For this review, take the finished solid that the model builds, in its own axes (mm). Face numbers are marked on the shaded views. Coordinates: 2 decimals unless noted, no trailing zeros. Write each loop counter-clockwise with the first axis right and the second up, starting at its lowest first coordinate (ties: lowest second). Pieces come first, ordered by that corner, then holes.
1) To check wall thickness, follow line 1 along Z through (x, y) = (-60.9, 18); line 2 along X through (y, z) = (23, -2.5); line 3 along X through (y, z) = (-1, -20). State the ranges of each line that lie inside material, in increasing order.
2) We need section D-D on y = 45.5. Write out the cut boundary in (x, z), then the cut area to 3 significant figures.
3) We need section B-B on z = 20. Write out the cut boundary in (x, y).
4) We need section C-C on y = 6.5. Write out the cut boundary in (x, z), then the cut area to 3 significant figures.
5) We need section A-A on x = 45. Write out the cut boundary in (y, z), then the cut area to 4 significant figures.
6) Mouldability with a two-part tool opening along X and no side actions: class the marked faces 1, 2, 3 and 4 as pulls with the +X half, pulls with the -X half, needs draft (parallel to the pull), parting line crosses it, or undercut.
7) Insertion check: P1, Ø3, axis at x = -32.5, z = -2.5, coming from the +Y side; P2, Ø4, axis at y = 18, z = 20, coming from the -X side; P3, Ø2.5, axis at x = -61, z = 10, coming from the +Y side. Each pin has a flat end and moves straight along its axis. Give the tip position at first contact, or say it passes through.
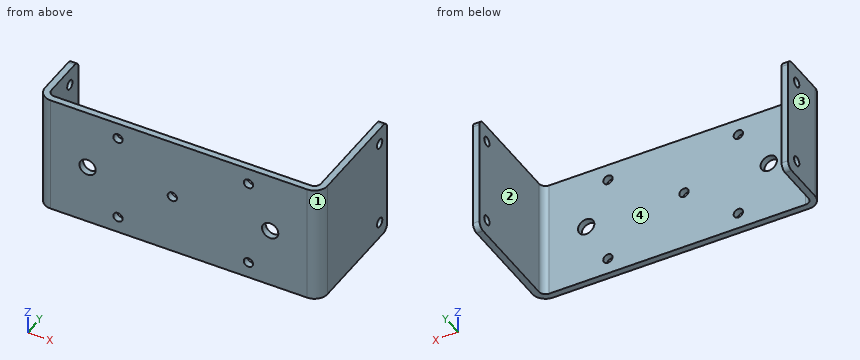
from build123d import *

# Parameters (mm, degrees)
SKETCH1_W                    = 124
SKETCH1_H                    = 55
SKETCH1_R                    = 1
SKETCH1_R_2                  = 3.75
BASE_FLANGE1_DEPTH           = 3
EDGE_FLANGE1_STRIP_W         = 18
EDGE_FLANGE1_STRIP_H         = 3
EDGE_FLANGE1_STRIP_CUT_DEPTH = 55
EDGE_FLANGE1_DEPTH           = 55
EDGE_FLANGE1_START           = 3
EDGE_FLANGE1_PROFILE_W       = 55
EDGE_FLANGE1_PROFILE_H       = 22
EDGE_FLANGE1_PROFILE_R       = 1
EDGE_FLANGE1_FLAT_DEPTH      = 3
EDGE_FLANGE2_STRIP_W         = 18
EDGE_FLANGE2_STRIP_H         = 3
EDGE_FLANGE2_STRIP_CUT_DEPTH = 55
EDGE_FLANGE2_DEPTH           = 55
EDGE_FLANGE2_START           = 3
EDGE_FLANGE2_PROFILE_W       = 55
EDGE_FLANGE2_PROFILE_H       = 48.5
EDGE_FLANGE2_PROFILE_R       = 1
EDGE_FLANGE2_FLAT_DEPTH      = 3
M4_CLEARANCE_HOLE1_D         = 4.3
M4_CLEARANCE_HOLE1_DEPTH     = 130
M4_CLEARANCE_HOLE2_D         = 4.3
M4_CLEARANCE_HOLE2_DEPTH     = 3
M4_CLEARANCE_HOLE2_TIP       = 1.291850331
M4_CLEARANCE_HOLE3_D         = 4.3
M4_CLEARANCE_HOLE3_DEPTH     = 3
M4_CLEARANCE_HOLE3_TIP       = 1.291850331
FILLET1_R                    = 3


# Sheet-metal steps are written as plain solids
with BuildPart() as part:
    # Sketch1 → Base-Flange1 (new body)
    with BuildSketch(Plane(origin=(0, 0, 0), x_dir=(1, 0, 0), z_dir=(0, 1, 0))):
        with Locations((3, 0)):
            Rectangle(SKETCH1_W, SKETCH1_H)
        with Locations(Location((-25, 20, 0), (0, 0, 270))):
            Circle(SKETCH1_R, mode=Mode.SUBTRACT)
        with Locations(Location((35, 20, 0), (0, 0, 270))):
            Circle(SKETCH1_R, mode=Mode.SUBTRACT)
        with Locations(Location((-25, -20, 0), (0, 0, 270))):
            Circle(SKETCH1_R, mode=Mode.SUBTRACT)
        with Locations(Location((35, -20, 0), (0, 0, 270))):
            Circle(SKETCH1_R, mode=Mode.SUBTRACT)
        with Locations(Location((45, 0, 0), (0, 0, 270))):
            Circle(SKETCH1_R_2, mode=Mode.SUBTRACT)
        with Locations(Location((-39, 0, 0), (0, 0, 270))):
            Circle(SKETCH1_R_2, mode=Mode.SUBTRACT)
        with Locations(Location((0, 0, 0), (0, 0, 270))):
            Circle(SKETCH1_R, mode=Mode.SUBTRACT)
    extrude(amount=-BASE_FLANGE1_DEPTH)

    # Edge-Flange1 strip (across the edge) → Edge-Flange1 strip cut (cut)
    with BuildSketch(Plane(origin=(-59, 0, -27.5), x_dir=(1, 0, 0), z_dir=(0, 0, 1))):
        with Locations((-6, -1.5)):
            Rectangle(EDGE_FLANGE1_STRIP_W, EDGE_FLANGE1_STRIP_H)
    extrude(amount=EDGE_FLANGE1_STRIP_CUT_DEPTH, mode=Mode.SUBTRACT)

    # Edge-Flange1 bend section (across the edge) → Edge-Flange1 (add)
    with BuildSketch(Plane(origin=(-59, 0, -27.5), x_dir=(1, 0, 0), z_dir=(0, 0, 1))):
        with BuildLine():
            Line((-3, 3), (0, 3))
            ThreePointArc((0, 3), (0.878679656, 0.878679656), (3, 0))
            Line((3, 0), (3, -3))
            ThreePointArc((3, -3), (-1.242640687, -1.242640687), (-3, 3))
        make_face()
    extrude(amount=EDGE_FLANGE1_DEPTH)

    # Edge-Flange1 profile (on flange) → Edge-Flange1 flat (add)
    with BuildSketch(Plane.ZY.offset(59).offset(EDGE_FLANGE1_START)):
        with Locations((0, 14)):
            Rectangle(EDGE_FLANGE1_PROFILE_W, EDGE_FLANGE1_PROFILE_H)
        with Locations((-20, 18)):
            Circle(EDGE_FLANGE1_PROFILE_R, mode=Mode.SUBTRACT)
        with Locations((20, 18)):
            Circle(EDGE_FLANGE1_PROFILE_R, mode=Mode.SUBTRACT)
    extrude(amount=-EDGE_FLANGE1_FLAT_DEPTH)

    # Edge-Flange2 strip (across the edge) → Edge-Flange2 strip cut (cut)
    with BuildSketch(Plane(origin=(65, 0, 27.5), x_dir=(-1, 0, 0), z_dir=(0, 0, -1))):
        with Locations((-6, -1.5)):
            Rectangle(EDGE_FLANGE2_STRIP_W, EDGE_FLANGE2_STRIP_H)
    extrude(amount=EDGE_FLANGE2_STRIP_CUT_DEPTH, mode=Mode.SUBTRACT)

    # Edge-Flange2 bend section (across the edge) → Edge-Flange2 (add)
    with BuildSketch(Plane(origin=(65, 0, 27.5), x_dir=(-1, 0, 0), z_dir=(0, 0, -1))):
        with BuildLine():
            Line((-3, 3), (0, 3))
            ThreePointArc((0, 3), (0.878679656, 0.878679656), (3, 0))
            Line((3, 0), (3, -3))
            ThreePointArc((3, -3), (-1.242640687, -1.242640687), (-3, 3))
        make_face()
    extrude(amount=EDGE_FLANGE2_DEPTH)

    # Edge-Flange2 profile (on flange) → Edge-Flange2 flat (add)
    with BuildSketch(Plane(origin=(65, 0, 0), x_dir=(0, 0, -1), z_dir=(1, 0, 0)).offset(EDGE_FLANGE2_START)):
        with Locations((0, 27.25)):
            Rectangle(EDGE_FLANGE2_PROFILE_W, EDGE_FLANGE2_PROFILE_H)
        with Locations((-20, 45.5)):
            Circle(EDGE_FLANGE2_PROFILE_R, mode=Mode.SUBTRACT)
        with Locations((20, 45.5)):
            Circle(EDGE_FLANGE2_PROFILE_R, mode=Mode.SUBTRACT)
    extrude(amount=-EDGE_FLANGE2_FLAT_DEPTH)

    # M4 Clearance Hole1
    with Locations(Plane(origin=(68, 0, 0), x_dir=(0, 0, -1), z_dir=(1, 0, 0))):
        with Locations((-20, 45.5), (20, 45.5)):
            Hole(M4_CLEARANCE_HOLE1_D / 2, depth=M4_CLEARANCE_HOLE1_DEPTH)

    # M4 Clearance Hole2
    with Locations(Plane.ZY.offset(62)):
        with Locations((-20, 18), (20, 18)):
            Hole(M4_CLEARANCE_HOLE2_D / 2, depth=M4_CLEARANCE_HOLE2_DEPTH)
            with Locations((0, 0, -(M4_CLEARANCE_HOLE2_DEPTH + M4_CLEARANCE_HOLE2_TIP / 2))):  # 118° drill point
                Cone(0, M4_CLEARANCE_HOLE2_D / 2, M4_CLEARANCE_HOLE2_TIP, mode=Mode.SUBTRACT)

    # M4 Clearance Hole3
    with Locations(Plane(origin=(0, -3, 0), x_dir=(-1, 0, 0), z_dir=(0, -1, 0))):
        with Locations((-35, 20), (25, 20), (25, -20), (-35, -20), (0, 0)):
            Hole(M4_CLEARANCE_HOLE3_D / 2, depth=M4_CLEARANCE_HOLE3_DEPTH)
            with Locations((0, 0, -(M4_CLEARANCE_HOLE3_DEPTH + M4_CLEARANCE_HOLE3_TIP / 2))):  # 118° drill point
                Cone(0, M4_CLEARANCE_HOLE3_D / 2, M4_CLEARANCE_HOLE3_TIP, mode=Mode.SUBTRACT)

    # Fillet1
    fillet1_edges = [part.edges().sort_by_distance(p)[0] for p in [
        (66.5, 51.5, 27.5),
        (66.5, 51.5, -27.5),
        (-60.5, 25, -27.5),
        (-60.5, 25, 27.5),
    ]]
    fillet(fillet1_edges, radius=FILLET1_R)


solid = part.part
Result:
1. line 1: z = -27.5 to -22.15, -17.85 to 17.85, 22.15 to 27.5
1. line 2: x = -62 to -59, 65 to 68
1. line 3: x = -60.47 to -27.15, -22.85 to 32.85, 37.15 to 66.47
2. outline: (65, -27.5) - (68, -27.5) - (68, -22.15) - (65, -22.15) - close; (65, -17.85) - (68, -17.85) - (68, 17.85) - (65, 17.85) - close; (65, 22.15) - (68, 22.15) - (68, 27.5) - (65, 27.5) - close
2. area: 139 mm2
3. outline: (-62, 3) arc R6 ccw to (-56, -3) - (-27.15, -3) - (-27.15, 0) - (-56, 0) arc R3 cw to (-59, 3) - (-59, 15.85) - (-62, 15.85) - close; (-62, 20.15) - (-59, 20.15) - (-59, 25) - (-62, 25) - close; (-22.85, -3) - (32.85, -3) - (32.85, 0) - (-22.85, 0) - close; (37.15, -3) - (62, -3) arc R6 ccw to (68, 3) - (68, 43.35) - (65, 43.35) - (65, 3) arc R3 cw to (62, 0) - (37.15, 0) - close; (65, 47.65) - (68, 47.65) - (68, 51.5) - (65, 51.5) - close
4. outline: (-62, -27.5) - (-59, -27.5) - (-59, 27.5) - (-62, 27.5) - close; (65, -27.5) - (68, -27.5) - (68, 27.5) - (65, 27.5) - close
4. area: 330 mm2
5. outline: (-3, -27.5) - (0, -27.5) - (0, -3.75) - (-3, -3.75) - close; (-3, 3.75) - (0, 3.75) - (0, 27.5) - (-3, 27.5) - close
5. area: 142.5 mm2
6. face 1: pulls with the +X half
6. face 2: undercut
6. face 3: pulls with the -X half
6. face 4: undercut
7. P1: stops at y = 0
7. P2: stops at x = 65
7. P3: stops at y = 25
